For this review, take the finished solid that the model builds, in its own axes (mm). A direction names the side the tool comes from. Give positions to 0.01 mm unless a question says otherwise; leave off trailing zeros. Order: outer loops, then holes, each group sorted by start corner. A loop starts at its lowest first (then second) coordinate and runs counter-clockwise, first axis right, second up. Notation, with made-up numbers: M 78.5,-5.75 L 102.5,-5.75 A21 cw 102.5,16.25 Z; hole C -10,-16 d4. An arc over 180 degrees is marked long. Answer as CSV lines item,"result". Start each with the question number.
1. For line 1 along X through (y, z) = (4, 0); line 2 along X through (y, z) = (8.75, 0); line 3 along Z through (x, y) = (3, 6.5), list the stretches that pass through material, from the lowest coordinate up.
2. Mouldability with a two-part tool opening along X and no side actions: class faces 1 (the flat face through (-18, 15, -5)), 2 (the cylindrical face through (0.26, 2.46, -23.79)), 3 (the cylindrical face through (23.77, 2.46, -0.18)), 4 (the cylindrical face through (-24.397, 2.465, 12.69)) as pulls with the +X half, pulls with the -X half, needs draft (parallel to the pull), parting line crosses it, or undercut.
3. Clearance check with flat-ended pins moving along their axes: P1, Ø3, axis at x = -20, y = 6, coming from the +Z side; P2, Ø4, axis at y = 10.5, z = 11, coming from the -X side; P3, Ø6, axis at x = -9.5, y = 6.5, coming from the -Z side. State where each tip first meets the part, or that it passes through.
4. We need section B-B, the plane x = 0. Give the boundary of the cut face in (y, z).
5. We need section A-A, the plane z = 0. Give the boundary of the cut face in (x, y), and give its area (3 significant figures).
6. Machinability: for faces 5 (the flat face through (-22.3, 5, -4.2)), 6 (the cylindrical face through (-7.086, 7.605, 17.089)), which of the approach directions +Z, -Z, +X, -X, +Y, -Y give a long, thin tool a straight path to every point of the face, cutting with its end or side? Answer none if there is none.
7. We need section D-D, the plane y = 2.75. Give the boundary of the cut face in (x, z), and give its area (3 significant figures).
8. We need section C-C, the plane x = 11. Give the boundary of the cut face in (y, z), and give its area (3 significant figures).
from build123d import *

# Parameters (mm, degrees)
SKETCH_2_R          = 27.5
SKETCH_2_R_2        = 0.85
EXTRUDE_1_DEPTH     = 5
SKETCH_3_R          = 22.5
EXTRUDE_2_DEPTH     = 10
SKETCH_4_R          = 18.5
CUT_EXTRUDE_1_DEPTH = 42.683330001


with BuildPart() as part:
    # 草图2 → 凸台-拉伸1 (new body)
    with BuildSketch(Plane(origin=(0, 0, 0), x_dir=(1, 0, 0), z_dir=(0, 1, 0))):
        with Locations(Location((0, 0, 0), (0, 0, 270))):
            Circle(SKETCH_2_R)
        with Locations(Location((0, 24.6, 0), (0, 0, 270))):
            Circle(SKETCH_2_R_2, mode=Mode.SUBTRACT)
        with Locations(Location((24.6, 0, 0), (0, 0, 270))):
            Circle(SKETCH_2_R_2, mode=Mode.SUBTRACT)
        with Locations(Location((0, -24.6, 0), (0, 0, 270))):
            Circle(SKETCH_2_R_2, mode=Mode.SUBTRACT)
        with Locations(Location((-24.6, 0, 0), (0, 0, 270))):
            Circle(SKETCH_2_R_2, mode=Mode.SUBTRACT)
    extrude(amount=EXTRUDE_1_DEPTH)

    # 草图3 → 凸台-拉伸2 (add)
    with BuildSketch(Plane(origin=(0, 5, 0), x_dir=(1, 0, 0), z_dir=(0, 1, 0))):
        with Locations(Location((0, 0, 0), (0, 0, 270))):
            Circle(SKETCH_3_R)
    extrude(amount=EXTRUDE_2_DEPTH)

    # 草图4 → 切除-拉伸1 (cut, through all)
    with BuildSketch(Plane(origin=(0, 15, 0), x_dir=(1, 0, 0), z_dir=(0, 1, 0))):
        with Locations(Location((0, 0, 0), (0, 0, 270))):
            Circle(SKETCH_4_R)
    extrude(amount=-CUT_EXTRUDE_1_DEPTH, mode=Mode.SUBTRACT)


solid = part.part
Result set:
1,line 1,"-27.5 to -25.45, -23.75 to -18.5, 18.5 to 23.75, 25.45 to 27.5"
1,line 2,"-22.5 to -18.5, 18.5 to 22.5"
1,line 3,"-22.3 to -18.26, 18.26 to 22.3"
2,face 1,"needs draft"
2,face 2,"undercut"
2,face 3,"undercut"
2,face 4,"parting line crosses it"
3,P1,"z = 19.99"
3,P2,"x = -20.62"
3,P3,"z = -26.62"
4,outline,"M 0,-27.5 L 5,-27.5 L 5,-25.45 L 0,-25.45 Z; M 0,-23.75 L 5,-23.75 L 5,-22.5 L 15,-22.5 L 15,-18.5 L 0,-18.5 Z; M 0,18.5 L 15,18.5 L 15,22.5 L 5,22.5 L 5,23.75 L 0,23.75 Z; M 0,25.45 L 5,25.45 L 5,27.5 L 0,27.5 Z"
5,outline,"M -27.5,0 L -25.45,0 L -25.45,5 L -27.5,5 Z; M -23.75,0 L -18.5,0 L -18.5,15 L -22.5,15 L -22.5,5 L -23.75,5 Z; M 18.5,0 L 23.75,0 L 23.75,5 L 22.5,5 L 22.5,15 L 18.5,15 Z; M 25.45,0 L 27.5,0 L 27.5,5 L 25.45,5 Z"
5,area,"153 mm2"
6,face 5,"+Y"
6,face 6,"+Y, -Y"
7,outline,"C 0,0 d55; hole C -24.6,0 d1.7; hole C 0,0 d37; hole C 0,-24.6 d1.7; hole C 0,24.6 d1.7; hole C 24.6,0 d1.7"
7,area,"1,290 mm2"
8,outline,"M 0,-25.2 L 5,-25.2 L 5,-19.63 L 15,-19.63 L 15,-14.87 L 0,-14.87 Z; M 0,14.87 L 15,14.87 L 15,19.63 L 5,19.63 L 5,25.2 L 0,25.2 Z"
8,area,"198 mm2"
